Work out the finished part from the listing and answer in its coordinate system (mm). Coordinates: 2 decimals unless noted, no trailing zeros. Order: outer loops, then holes, each group sorted by start corner. A loop starts at its lowest first (then second) coordinate and runs counter-clockwise, first axis right, second up. Notation, with made-up numbers: M -35.75,-10.5 L -4.75,-10.5 A9 ccw -4.75,0.5 Z; hole C 17,-24.75 d10. An arc over 180 degrees is marked long. Write item = value, one per line. Start each with the question number.
Q1. Each of these flat-tipped pins is pushed along its axis until it touches: P1, Ø1.5, axis at y = -8, z = 1, coming from the +X side; P2, Ø1.5, axis at y = -5, z = 1, coming from the -X side; P3, Ø1.5, axis at x = 10, z = 1, coming from the -Y side; P4, Ø4, axis at x = 34.5, y = 17, coming from the -Z side. Where does it stop, or does it pass through?
Q2. Find section C-C on z = 1.7. Give the number of separate pieces and of enclosed holes in the cut face, and give its area (3 significant figures).
Q3. Find section A-A on x = 28. Give the vertices of the cut face in (y, z), and give its area (4 significant figures).
Q4. Straight lines are drawn through the part: line 1 along Y through (x, z) = (37, 0.7); line 2 along X through (y, z) = (24.5, 1.9); line 3 along Y through (x, z) = (7.5, 2.05). For each, find the intervals that lie inside material, in ascending order.
Q5. Find section B-B on y = -2.5. Give the vertices of the cut face in (x, z), and give its area (3 significant figures).
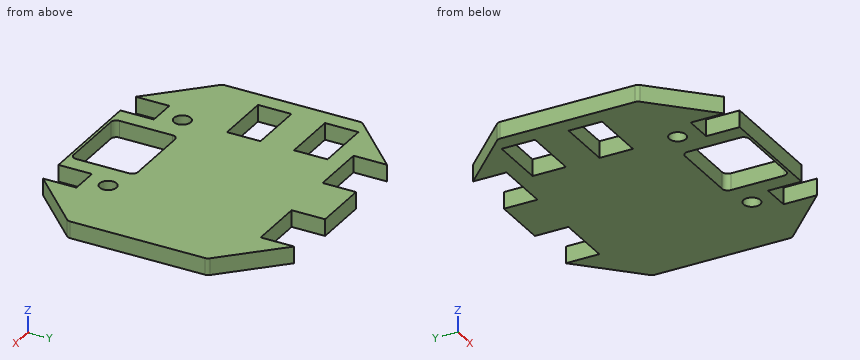
```python
from build123d import *

# Parameters (mm, degrees)
SKETCH1_R           = 1.5
SKETCH1_W           = 14
SKETCH1_H           = 11.5
BOSS_EXTRUDE1_DEPTH = 3
SKETCH2_W           = 10
SKETCH2_H           = 6
SKETCH2_W_2         = 5
CUT_EXTRUDE1_DEPTH  = 62.10646447
SKETCH3_W           = 10
SKETCH3_H           = 6
CUT_EXTRUDE2_DEPTH  = 62.10646447
FILLET1_R           = 1


with BuildPart() as part:
    # Sketch1 → Boss-Extrude1 (new body)
    with BuildSketch(Plane.XY):
        Polygon((0, 0), (0, 25), (10, 35), (40, 35), (50, 25), (50, 0), (40, -10), (10, -10), align=None)
        with Locations((13, 0)):
            Circle(SKETCH1_R, mode=Mode.SUBTRACT)
        with Locations((37, 0)):
            Circle(SKETCH1_R, mode=Mode.SUBTRACT)
        with Locations((25, -3.75)):
            Rectangle(SKETCH1_W, SKETCH1_H, mode=Mode.SUBTRACT)
    extrude(amount=BOSS_EXTRUDE1_DEPTH)

    # Sketch2 → Cut-Extrude1 (cut, through all)
    with BuildSketch(Plane.XY.offset(3)):
        with Locations((15, 32)):
            Rectangle(SKETCH2_W, SKETCH2_H)
        with Locations((35, 32)):
            Rectangle(SKETCH2_W, SKETCH2_H)
        with Locations((12.5, -7)):
            Rectangle(SKETCH2_W_2, SKETCH2_H)
        with Locations((37.5, -7)):
            Rectangle(SKETCH2_W_2, SKETCH2_H)
    extrude(amount=-CUT_EXTRUDE1_DEPTH, mode=Mode.SUBTRACT)

    # Sketch3 → Cut-Extrude2 (cut, through all)
    with BuildSketch(Plane.XY.offset(3)):
        with Locations((8, 11)):
            Rectangle(SKETCH3_W, SKETCH3_H)
        with Locations((8, 23)):
            Rectangle(SKETCH3_W, SKETCH3_H)
    extrude(amount=-CUT_EXTRUDE2_DEPTH, mode=Mode.SUBTRACT)

    # Fillet1
    fillet1_edges = [part.edges().sort_by_distance(p)[0] for p in [
        (0, 0, 1.5),
        (0, 25, 1.5),
        (50, 25, 1.5),
        (50, 0, 1.5),
        (18, 2, 1.5),
        (18, -9.5, 1.5),
        (32, -9.5, 1.5),
        (32, 2, 1.5),
    ]]
    fillet(fillet1_edges, radius=FILLET1_R)


solid = part.part
```
Findings below:
q1.P1 = 42.75
q1.P2 = 4.25
q1.P3 = -10
q1.P4 = 0
q2.separate_pieces = 1
q2.enclosed_holes = 5
q2.area = 1,580 mm^2
q3.outline = M -10,0 L -9.5,0 L -9.5,3 L -10,3 Z; M 2,0 L 35,0 L 35,3 L 2,3 Z
q3.area = 100.5 mm^2
q4.line_1 = -4 to -1.5, 1.5 to 29
q4.line_2 = 0 to 3, 13 to 50
q4.line_3 = -7.5 to 8, 14 to 20, 26 to 32.5
q5.outline = M 2.5,0 L 18,0 L 18,3 L 2.5,3 Z; M 32,0 L 47.5,0 L 47.5,3 L 32,3 Z
q5.area = 93.0 mm^2
